Geometry: final body of the model. Coordinates: model frame, mm. A direction names the side the tool comes from. Coordinates: 2 decimals unless noted, no trailing zeros. Order: outer loops, then holes, each group sorted by start corner. A loop starts at its lowest first (then second) coordinate and runs counter-clockwise, first axis right, second up. Notation, with made-up numbers: (-28.75, 88.5) -> (21.25, 88.5) arc R9 ccw to (21.25, 105.5) -> close; hole circle Ø8 at (33, 48). An arc over 180 degrees is marked (long way). Use one line per item in the form item = value.
Autodesk Inventor part; units mm, degrees
ref_plane "Work Plane1" through (0, 60, 0) normal (0, 1, 0) x (-1, 0, 0)
ref_plane "YZ Plane" through (0, 0, 0) normal (1, 0, 0) x (0, 1, 0)
ref_plane "XY Plane" through (0, 0, 0) normal (0, 0, 1) x (1, 0, 0)
sketch "Sketch1" plane through (0, 0, 0) normal (0, 1, 0) x (-1, 0, 0)
  line L0 (-60, -60) -> (60, -60)
  line L1 (60, -60) -> (60, 60)
  line L2 (60, 60) -> (-60, 60)
  line L3 (-60, 60) -> (-60, -60)
  line L4 (-60, -60) -> (60, 60) construction
  line L5 (60, -60) -> (-60, 60) construction
  circle A0 centre (0, 0) radius 56
  line L6 (0, 60) -> (0, 0) construction
  circle A1 centre (0, 0) radius 53
  point P0 (-52, 52)
  dimension "d0" = 120
  dimension "d1" = 120
  dimension "d2" = 112
  dimension "d4" = 104
  dimension "d29" = 3
extrude "Extrusion1" add sketch "Sketch1" against normal blind 3 contours L3 L2 L1 L0 | A0
hole "Hole1" at (52, 0, 52) direction (0, -1, 0) diameter 4.4 end through all
pattern_circular "Circular Pattern1" count 4 over 360 about axis through (0, -10, 0) along (0, 1, 0) of "Hole1"
ref_plane "Work Plane1" through (0, 60, 0) normal (0, 1, 0) x (-1, 0, 0)
sketch "Sketch3" plane through (0, 60, 0) normal (0, 1, 0) x (-1, 0, 0)
  circle A0 centre (0, 0) radius 48.26
  circle A1 centre (0, 0) radius 45.26
  dimension "d21" = 96.52
  dimension "WallThickness" = 3
loft "Loft1" add profiles "Sketch3", "Sketch1" contours A0 | A1 / A0 | A1
loft "Loft2" cut profiles "Sketch1", "Sketch3" contours A1 / A1
fillet "Fillet1" radius 2 3 edges at (56, 0, 0) (53, 0, 0) (53, -3, 0)
fillet "Fillet2" radius 1.5 2 edges at (48.26, 60, 0) (45.26, 60, 0)
equation "\"d29\" = WallThickness"
equation "\"d36\" = 0.5 * WallThickness"
properties part number "120mm-4in duct adapter"
1) Pull-direction query (Z, two-part tool) for faces 3 (the flat face through (1, -1, -60)), 4 (the flat face through (31, 0, 49)), 5 (the cylindrical face through (50.254, -1.521, -53.339)); classes: released by +Z, released by -Z, zero draft, split by the parting line, or undercut.
Results found:
face_3 = released by -Z
face_4 = zero draft
face_5 = undercut
2) Section A-A, the plane y = 14. Output: boundary loops of the cut face in (x, z).
Results found:
outline = circle Ø108.39 at (0, 0); hole circle Ø102.39 at (0, 0)
3) Material intervals for probe 1 along Z at (x, y) = (0, -0.45); probe 2 along X at (y, z) = (31, 25.5); probe 3 along Z at (x, y) = (32.5, 27.5), sorted ascending. Write a range as from..to.
Results found:
probe_1 = -60..-53, 53..60
probe_2 = -45.32..-41.84, 41.84..45.32
probe_3 = -41.17..-37.27, 37.27..41.17
4) Access query for faces 1 (the cylindrical face through (-53.339, -1.521, -50.254)), 2 (the cylindrical face through (-28.49, -0.56, 44.69)). Directions: +Z, -Z, +X, -X, +Y, -Y. A direction counts if a zero-diameter tool reaches every point of the face in a straight line with its end or side. Return the directions, or none.
Results found:
face_1 = +Y, -Y
face_2 = -Y
5) Contact query for flat-ended pins moving along their axis: P1, Ø1, axis at y = 10, z = -14, coming from the -X side; P2, Ø5, axis at y = 29, z = 26.5, coming from the -X side; P3, Ø7, axis at x = 52, z = 52, coming from the +Y side. Output: stop coordinate, or through.
Results found:
P1 = -53.03
P2 = -46.47
P3 = 0
6) Section B-B, the plane y = 45. Output: boundary loops of the cut face in (x, z) (3 decimals).
Results found:
outline = circle Ø100.39 at (0, 0); hole circle Ø94.39 at (0, 0)
